Geometry: final body of the model. Coordinates: model frame, mm. A direction names the side the tool comes from. Give positions to 0.01 mm unless a question says otherwise; leave off trailing zeros. Order: outer loops, then holes, each group sorted by start corner. A loop starts at its lowest first (then second) coordinate and runs counter-clockwise, first axis right, second up. Notation, with made-up numbers: (17, -31) -> (37, -31) arc R24 ccw to (37, -12) -> close; hole circle Ø4 at (28, 39). An arc over 180 degrees is marked (long way). One line per question, with ' | ' between items. Start each with the question number.
(1) Section C-C (x = 28.5). Return loops of the section in (y, z), then the cut area to 3 significant figures.
(2) Section A-A (x = -27.5). Return loops of the section in (y, z).
(3) First-contact query: pin 1 Ø9 at (x, y) = (-10, 7) entering from -Z; pin 2 Ø4 at (x, z) = (2, -2.5) entering from -Y; pin 3 Ø2.5 at (y, z) = (-10, -4) entering from -X; pin 4 Ø2.5 at (y, z) = (10, -4) entering from +X. Flat tips, straight axial feed; report the tip coordinate or a pass-through.
(4) Ray query, L1, parallel to X at y = -8, z = -4.5; L2, parallel to X at y = 4.25, z = -0.25; L3, parallel to X at y = 0.5, z = -3. Return the intervals inside material, ascending.
(5) Set-up query: faces 4 (the face through (35.979, 9.425, -2.614)), 5 (the face through (15, 8, -6)), 6 (the face through (19.478, -3.553, -0.119)), 7 (the face through (14.07, 7.43, 1.78)), 8 (the face through (0, -15, 1)). Return all of +Z, -Z, +X, -X, +Y, -Y with unobstructed straight access to the full face (end or side cutting, diameter ignored); none if empty.
(6) Section B-B (y = -6). Return loops of the section in (x, z), then the cut area to 3 significant figures.
(7) Mould query, pull axis Y, two halves, no side actions, for faces 1 (the face through (36, 0, -7)), 2 (the face through (-29, 0, 2)), 3 (the face through (15.4, -12.5, -3.5)). Classes: +Y half, -Y half, draft (parallel to the pull), parting line (faces both ways), or undercut.
```python
from build123d import *

# Parameters (mm, degrees)
SKETCH1_W               = 75
SKETCH1_H               = 30
BOSS_EXTRUDE1_DEPTH     = 3
SKETCH2_W               = 3
SKETCH2_H               = 30
BOSS_EXTRUDE2_DEPTH     = 7
SKETCH4_R               = 1.5
CUT_EXTRUDE1_DEPTH      = 3
MIRROR1_COPY_1_SKETCH_R = 1.5
MIRROR1_COPY_1_DEPTH    = 3
SKETCH5_W               = 16
SKETCH5_H               = 7
BOSS_EXTRUDE3_DEPTH     = 8
CHAMFER1_SIZE           = 5
CHAMFER1_SIZE2          = 7
CHAMFER2_SIZE           = 5
CHAMFER3_SIZE           = 2
SKETCH6_R               = 1.5
CUT_EXTRUDE2_DEPTH      = 8
CUT_EXTRUDE3_START      = -5
CUT_EXTRUDE3_DEPTH      = 42.149507332
CHAMFER4_SIZE           = 7
CHAMFER4_SIZE2          = 5
CHAMFER5_SIZE           = 5
CHAMFER6_SIZE           = 2
SKETCH8_R               = 1.5
CUT_EXTRUDE4_DEPTH      = 42.608292443


with BuildPart() as part:
    # Sketch1 → Boss-Extrude1 (new body)
    with BuildSketch(Plane.XY):
        Rectangle(SKETCH1_W, SKETCH1_H)
    extrude(amount=BOSS_EXTRUDE1_DEPTH)

    # Sketch2 → Boss-Extrude2 (add)
    with BuildSketch(Plane(origin=(0, 0, 0), x_dir=(-1, 0, 0), z_dir=(0, 0, -1))):
        with Locations((-36, 0)):
            Rectangle(SKETCH2_W, SKETCH2_H)
    boss_extrude2 = extrude(amount=BOSS_EXTRUDE2_DEPTH)

    # Sketch4 → Cut-Extrude1 (cut)
    with BuildSketch(Plane.ZY.offset(-34.5)):
        with Locations((-4, 10)):
            Circle(SKETCH4_R)
    cut_extrude1 = extrude(amount=-CUT_EXTRUDE1_DEPTH, mode=Mode.SUBTRACT)

    # Mirror2: Cut-Extrude1 across plane
    add(cut_extrude1.mirror(Plane.ZX), mode=Mode.SUBTRACT)

    # Mirror1: Boss-Extrude2, Cut-Extrude1 across plane
    add(boss_extrude2.mirror(Plane(origin=(0, 0, 0), x_dir=(0, 0, 1), z_dir=(1, 0, 0))))
    add(cut_extrude1.mirror(Plane(origin=(0, 0, 0), x_dir=(0, 0, 1), z_dir=(1, 0, 0))), mode=Mode.SUBTRACT)

    # Mirror1 copy 1 sketch → Mirror1 copy 1 (cut)
    with BuildSketch(Plane(origin=(-34.5, 0, 0), x_dir=(0, 0, 1), z_dir=(1, 0, 0))):
        with Locations((-4, 10)):
            Circle(MIRROR1_COPY_1_SKETCH_R)
    extrude(amount=-MIRROR1_COPY_1_DEPTH, mode=Mode.SUBTRACT)

    # Sketch5 → Boss-Extrude3 (add)
    with BuildSketch(Plane.XZ.offset(15)):
        with Locations((15.5, -3.5)):
            Rectangle(SKETCH5_W, SKETCH5_H)
    boss_extrude3 = extrude(amount=-BOSS_EXTRUDE3_DEPTH)

    # Chamfer1
    chamfer1_edges = [part.edges().sort_by_distance(p)[0] for p in [
        (15.5, -15, -7),
    ]]
    chamfer1_side = [part.faces().sort_by_distance(p)[0] for p in [
        (15.5, -11, -7),
    ]]
    chamfer(chamfer1_edges, length=CHAMFER1_SIZE, length2=CHAMFER1_SIZE2, reference=chamfer1_side[0])

    # Chamfer2
    chamfer2_edges = [part.edges().sort_by_distance(p)[0] for p in [
        (15.5, -7, 0),
    ]]
    chamfer(chamfer2_edges, length=CHAMFER2_SIZE)

    # Chamfer3
    chamfer3_edges = [part.edges().sort_by_distance(p)[0] for p in [
        (15.5, -7, -7),
    ]]
    chamfer(chamfer3_edges, length=CHAMFER3_SIZE - 0.0001)  # a hair under: the kernel refuses the full size

    # Sketch6 → Cut-Extrude2 (cut)
    with BuildSketch(Plane(origin=(0, -9.932432432, -7.094594595), x_dir=(1, 0, 0), z_dir=(0, -0.8137334712067358, -0.5812381937190955))):
        with Locations(Location((11.5, 4.718572906, 0), (0, 0, 270))):
            Circle(SKETCH6_R)
        with Locations(Location((19.5, 4.718572906, 0), (0, 0, 270))):
            Circle(SKETCH6_R)
    cut_extrude2 = extrude(amount=-CUT_EXTRUDE2_DEPTH, mode=Mode.SUBTRACT)

    # Sketch7 → Cut-Extrude3 (cut, through all)
    with BuildSketch(Plane(origin=(0, -9.932432432, -7.094594595), x_dir=(1, 0, 0), z_dir=(0, -0.8137334712067358, -0.5812381937190955)).offset(CUT_EXTRUDE3_START)):
        Polygon((8.324573519, 4.718572906), (9.91228676, 1.968572906), (13.08771324, 1.968572906), (14.675426481, 4.718572906), (13.08771324, 7.468572906), (9.91228676, 7.468572906), align=None)
        Polygon((16.324573519, 4.718572906), (17.91228676, 1.968572906), (21.08771324, 1.968572906), (22.675426481, 4.718572906), (21.08771324, 7.468572906), (17.91228676, 7.468572906), align=None)
    cut_extrude3 = extrude(amount=-CUT_EXTRUDE3_DEPTH, mode=Mode.SUBTRACT)

    # Mirror3: Boss-Extrude3 across plane
    add(boss_extrude3.mirror(Plane.ZX))

    # Chamfer4
    chamfer4_edges = [part.edges().sort_by_distance(p)[0] for p in [
        (15.5, 15, -7),
    ]]
    chamfer4_side = [part.faces().sort_by_distance(p)[0] for p in [
        (0, 15, 2.243362702),
    ]]
    chamfer(chamfer4_edges, length=CHAMFER4_SIZE, length2=CHAMFER4_SIZE2, reference=chamfer4_side[0])

    # Chamfer5
    chamfer5_edges = [part.edges().sort_by_distance(p)[0] for p in [
        (15.5, 7, 0),
    ]]
    chamfer(chamfer5_edges, length=CHAMFER5_SIZE)

    # Chamfer6
    chamfer6_edges = [part.edges().sort_by_distance(p)[0] for p in [
        (15.5, 7, -7),
    ]]
    chamfer(chamfer6_edges, length=CHAMFER6_SIZE - 0.0001)  # a hair under: the kernel refuses the full size

    # Mirror4: Cut-Extrude2, Cut-Extrude3 across plane
    add(cut_extrude2.mirror(Plane.ZX), mode=Mode.SUBTRACT)
    add(cut_extrude3.mirror(Plane.ZX), mode=Mode.SUBTRACT)

    # Sketch8 → Cut-Extrude4 (cut, through all)
    with BuildSketch(Plane.XY.offset(3)):
        with Locations((-27.5, 0)):
            Circle(SKETCH8_R)
    extrude(amount=-CUT_EXTRUDE4_DEPTH, mode=Mode.SUBTRACT)


solid = part.part
```
Response:
1) outline: (-15, 0) -> (15, 0) -> (15, 3) -> (-15, 3) -> close | area: 90.0 mm^2
2) outline: (-15, 0) -> (-1.5, 0) -> (-1.5, 3) -> (-15, 3) -> close; (1.5, 0) -> (15, 0) -> (15, 3) -> (1.5, 3) -> close
3) pin 1: stops at z = 0 | pin 2: passes through | pin 3: stops at x = 7.5 | pin 4: stops at x = 23.5
4) L1: x = -37.5 to -34.5, 7.5 to 23.5, 34.5 to 37.5 | L2: x = -37.5 to -34.5, 7.5 to 9.74, 13.26 to 17.74, 21.26 to 23.5, 34.5 to 37.5 | L3: x = -37.5 to -34.5, 34.5 to 37.5
5) face 4: +X | face 5: -Z | face 6: +Z | face 7: none | face 8: +Z, -Z, +X, -X, -Y
6) outline: (-37.5, -7) -> (-34.5, -7) -> (-34.5, 0) -> (7.5, 0) -> (7.5, -4) -> (23.5, -4) -> (23.5, 0) -> (34.5, 0) -> (34.5, -7) -> (37.5, -7) -> (37.5, 3) -> (21.98, 3) -> (22.68, 1.51) -> (21.09, -1.87) -> (17.91, -1.87) -> (16.32, 1.51) -> (17.02, 3) -> (13.98, 3) -> (14.68, 1.51) -> (13.09, -1.87) -> (9.91, -1.87) -> (8.32, 1.51) -> (9.02, 3) -> (-37.5, 3) -> close | area: 282 mm^2
7) face 1: draft | face 2: undercut | face 3: -Y half
